Source: CAD feature listing. Evaluate the final solid. Frame: model axes, mm. A direction names the side the tool comes from. Give positions to 0.01 mm unless a question says otherwise; leave off trailing zeros. Write each loop counter-clockwise with the first axis right and the second up, starting at its lowest first coordinate (ties: lowest second). Pieces come first, ordered by that corner, then holes. Notation, with made-up numbers: M 19,28.5 L 48,28.5 A11 cw 48,47.5 Z; hole C 20,-26.75 d9. An arc over 180 degrees is marked long. Return JSON: item names as keys, results as strings.
```python
from build123d import *

# Parameters (mm, degrees)
BOSS_EXTRUDE1_DEPTH = 4
SKETCH4_R           = 10
BOSS_EXTRUDE2_DEPTH = 3
CUT_EXTRUDE3_DEPTH  = 11
SKETCH5_R           = 2.5
BOSS_EXTRUDE4_DEPTH = 9


with BuildPart() as part:
    # Sketch3 → Boss-Extrude1 (new body)
    with BuildSketch(Plane.XY):
        with BuildLine():
            Line((-10, 0), (-5, 100))
            ThreePointArc((-5, 100), (0, 105), (5, 100))
            Line((5, 100), (10, 0))
            ThreePointArc((10, 0), (0, -10), (-10, 0))
        make_face()
    extrude(amount=BOSS_EXTRUDE1_DEPTH)

    # Sketch4 → Boss-Extrude2 (add)
    with BuildSketch(Plane.XY.offset(4)):
        Circle(SKETCH4_R)
    extrude(amount=BOSS_EXTRUDE2_DEPTH)

    # Sketch2 → Cut-Extrude3 (cut)
    with BuildSketch(Plane.XY):
        with BuildLine():
            Line((-2, -1.5), (2, -1.5))
            ThreePointArc((2, -1.5), (2.5, 0), (2, 1.5))
            Line((2, 1.5), (-2, 1.5))
            ThreePointArc((-2, 1.5), (-2.5, 0), (-2, -1.5))
        make_face()
    extrude(amount=CUT_EXTRUDE3_DEPTH, mode=Mode.SUBTRACT)

    # Sketch5 → Boss-Extrude4 (add)
    with BuildSketch(Plane.XY.offset(4)):
        with Locations((0, 100)):
            Circle(SKETCH5_R)
    extrude(amount=-BOSS_EXTRUDE4_DEPTH)


solid = part.part
```
1) Set-up query: faces 4 (the face through (-0.33, 102.48, -2.46)), 5 (the face through (-2.17, -9.76, 4.23)), 6 (the face through (2.5, 0, 3.5)). Return all of +Z, -Z, +X, -X, +Y, -Y with unobstructed straight access to the full face (end or side cutting, diameter ignored); none if empty.
Numbers:
{"face 4": "-Z", "face 5": "+Z", "face 6": "+Z, -Z"}
2) Cut plane A-A, the plane x = 0. Return the cut outline in (y, z).
Numbers:
{"outline": "M -10,0 L -1.5,0 L -1.5,7 L -10,7 Z; M 1.5,0 L 97.5,0 L 97.5,-5 L 102.5,-5 L 102.5,0 L 105,0 L 105,4 L 10,4 L 10,7 L 1.5,7 Z"}
3) Draft query along X for faces 1 (the face through (0, 1.5, 3)), 2 (the face through (0, 54, 4)), 3 (the face through (7.465, 50.7, 1.972)). Return one class per face: released by +X, released by -X, zero draft, split by the parting line, or undercut.
Numbers:
{"face 1": "undercut", "face 2": "zero draft", "face 3": "released by +X"}
4) Contact query for flat-ended pins moving along their axis: pin 1 Ø10 at (x, y) = (-2, 72) entering from -Z; pin 2 Ø4 at (x, z) = (-3.5, 4.5) entering from -Y; pin 3 Ø5 at (x, z) = (-7, 1.5) entering from +Y. Output: stop coordinate, or through.
Numbers:
{"pin 1": "stops at z = 0", "pin 2": "stops at y = -9.89", "pin 3": "stops at y = 102.18"}
5) Cut plane B-B, the plane z = 1. Return the cut outline in (x, y), then the cut area to 3 significant figures.
Numbers:
{"outline": "M -10,0 A10 ccw 10,0 L 5,100 A5 ccw -5,100 Z; hole M -2,-1.5 L 2,-1.5 A2.5 ccw 2,1.5 L -2,1.5 A2.5 ccw Z", "area": "1,680 mm²"}
6) Cut plane D-D, the plane x = -6.75. Return the cut outline in (y, z), then the cut area to 3 significant figures.
Numbers:
{"outline": "M -7.38,0 L 65,0 L 65,4 L 7.38,4 L 7.38,7 L -7.38,7 Z", "area": "334 mm²"}
7) Line query: line 1 (Z direction, x = -5.5, y = 84.5); line 2 (X direction, y = 44, z = 1); line 3 (X direction, y = 68, z = 1.75). Output: solid intervals per line, ascending. Write a range as [from, to].
Numbers:
{"line 1": "z = [0, 4]", "line 2": "x = [-7.8, 7.8]", "line 3": "x = [-6.6, 6.6]"}
8) Cut plane C-C, the plane y = 20. Return the cut outline in (x, z).
Numbers:
{"outline": "M -9,0 L 9,0 L 9,4 L -9,4 Z"}
